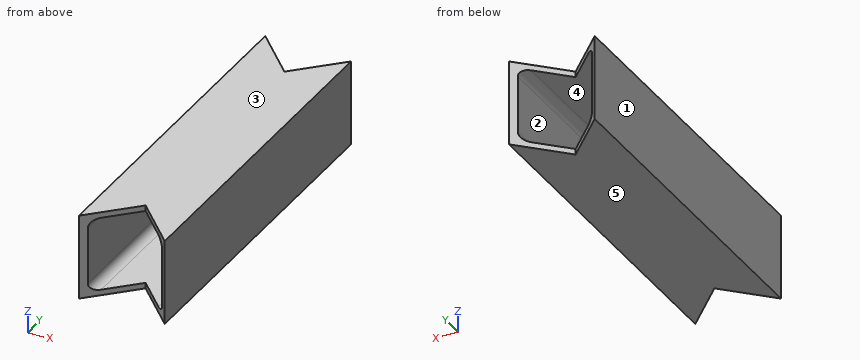
from build123d import *

# Parameters (mm, degrees)
BOSS_EXTRU_1_DEPTH      = 30
ENL_V_MAT_EXTRU_1_DEPTH = 171


with BuildPart() as part:
    # Esquisse1 → Boss.-Extru.1 (new body)
    with BuildSketch(Plane.XY):
        Polygon((0, 0), (0, 117.56958174), (15, 102.56958174), (30, 117.56958174), (30, 0), (15, 15), align=None)
    extrude(amount=BOSS_EXTRU_1_DEPTH)

    # Esquisse2 → Enlèv. mat.-Extru.1 (cut)
    with BuildSketch(Plane(origin=(0, 0, 0), x_dir=(1, 0, 0), z_dir=(0, 1, 0))):
        with BuildLine():
            Line((5, -28), (25, -28))
            ThreePointArc((25, -28), (27.121320344, -27.121320344), (28, -25))
            Line((28, -25), (28, -5))
            ThreePointArc((28, -5), (27.121320344, -2.878679656), (25, -2))
            Line((25, -2), (5, -2))
            ThreePointArc((5, -2), (2.878679656, -2.878679656), (2, -5))
            Line((2, -5), (2, -25))
            ThreePointArc((2, -25), (2.878679656, -27.121320344), (5, -28))
        make_face()
    extrude(amount=ENL_V_MAT_EXTRU_1_DEPTH, mode=Mode.SUBTRACT)


solid = part.part
CAD build for the part. Positions are in the model's coordinates, mm. Face numbers are marked on the shaded views. A direction names the side the tool comes from. Round coordinates to 2 decimals unless told otherwise and drop trailing zeros. Write each loop counter-clockwise with the first axis right and the second up, starting at its lowest first coordinate (ties: lowest second). Pieces come first, ordered by that corner, then holes.
(1) Slice it at D-D, the plane y = 63.5. Write the cut outline in (x, z), and give its area (3 significant figures).
(2) 3-axis set-ups, long thin cutter, end or side, ignore diameter. For the marked faces 4 and 5: which of +Z, -Z, +X, -X, +Y, -Y reach the whole face in a straight line?
(3) Mould opens along Z. For the marked faces 1, 2 and 3 say: pulls with the +Z half, pulls with the -Z half, needs draft (parallel to the pull), parting line crosses it, or undercut.
(4) Drop a flat-ended pin along its axis: P1, Ø12, axis at x = 6, y = 105.5, coming from the -Z side. Give the stop position or say it passes through.
(5) Probe line 1 along X through (y, z) = (50, 24); line 2 along X through (y, z) = (29, 27.5). List the from-to ranges inside material, lowest first.
(6) Slice it at A-A, the plane z = 17.5. Write the cut outline in (x, y).
(7) Slice it at C-C, the plane x = 6.25. Write the cut outline in (y, z), and give its area (3 significant figures).
(8) Slice it at B-B, the plane y = 7. Write the cut outline in (x, z).
From the geometry:
1. outline: (0, 0) - (30, 0) - (30, 30) - (0, 30) - close; hole (2, 5) arc R3 ccw to (5, 2) - (25, 2) arc R3 ccw to (28, 5) - (28, 25) arc R3 ccw to (25, 28) - (5, 28) arc R3 ccw to (2, 25) - close
1. area: 232 mm2
2. face 4: +Y, -Y
2. face 5: -Z, +X, -X, +Y, -Y
3. face 1: needs draft
3. face 2: undercut
3. face 3: pulls with the +Z half
4. P1: stops at z = 0
5. line 1: x = 0 to 2, 28 to 30
5. line 2: x = 0 to 3.34, 26.66 to 30
6. outline: (0, 0) - (2, 2) - (2, 115.57) - (0, 117.57) - close; (28, 2) - (30, 0) - (30, 117.57) - (28, 115.57) - close
7. outline: (6.25, 0) - (111.32, 0) - (111.32, 2) - (6.25, 2) - close; (6.25, 28) - (111.32, 28) - (111.32, 30) - (6.25, 30) - close
7. area: 420 mm2
8. outline: (0, 0) - (7, 0) - (7, 2) - (5, 2) arc R3 cw to (2, 5) - (2, 25) arc R3 cw to (5, 28) - (7, 28) - (7, 30) - (0, 30) - close; (23, 0) - (30, 0) - (30, 30) - (23, 30) - (23, 28) - (25, 28) arc R3 cw to (28, 25) - (28, 5) arc R3 cw to (25, 2) - (23, 2) - close
